The listing builds one solid part. Answer for the finished solid, in the listing's coordinates (mm). A direction names the side the tool comes from. Coordinates: 2 decimals unless noted, no trailing zeros. Write each loop counter-clockwise with the first axis right and the second up, starting at its lowest first coordinate (ties: lowest second). Pieces come first, ordered by that corner, then holes.
from build123d import *

# Parameters (mm, degrees)
SKETCH1_W           = 305
SKETCH1_H           = 305
BOSS_EXTRUDE2_DEPTH = 874
SKETCH3_W           = 100
SKETCH3_H           = 100
BOSS_EXTRUDE4_DEPTH = 100
CUT_EXTRUDE3_DEPTH  = 100
SKETCH8_W           = 305
SKETCH8_H           = 305
BOSS_EXTRUDE5_DEPTH = 66


with BuildPart() as part:
    # Sketch1 → Boss-Extrude2 (new body)
    with BuildSketch(Plane.XY):
        with Locations((152.5, 152.5)):
            Rectangle(SKETCH1_W, SKETCH1_H)
    extrude(amount=BOSS_EXTRUDE2_DEPTH)

    # Sketch3 → Boss-Extrude4 (add)
    with BuildSketch(Plane.ZY):
        with Locations((774, 152.5)):
            Rectangle(SKETCH3_W, SKETCH3_H)
    extrude(amount=BOSS_EXTRUDE4_DEPTH)

    # Sketch5 → Cut-Extrude3 (cut)
    with BuildSketch(Plane.XZ.offset(-102.5)):
        Polygon((-100, 824), (0, 824), (-100, 724), align=None)
    extrude(amount=-CUT_EXTRUDE3_DEPTH, mode=Mode.SUBTRACT)

    # Sketch2 → Cut-Loft2 section 0
    with BuildSketch(Plane(origin=(0, 0, 0), x_dir=(-1, 0, 0), z_dir=(0, 0, -1))):
        with BuildLine():
            Line((-242.5, 242.5), (-62.5, 242.5))
            Line((-62.5, 242.5), (-62.5, 62.5))
            Line((-62.5, 62.5), (-242.5, 62.5))
            Line((-242.5, 62.5), (-242.5, 242.5))
        make_face()
    # Sketch6 → Cut-Loft2 section 1
    with BuildSketch(Plane.XY.offset(874)):
        with BuildLine():
            Line((22.5, 282.5), (282.5, 282.5))
            Line((282.5, 282.5), (282.5, 22.5))
            Line((282.5, 22.5), (22.5, 22.5))
            Line((22.5, 22.5), (22.5, 282.5))
        make_face()
    loft(mode=Mode.SUBTRACT)

    # Sketch8 → Boss-Extrude5 (add)
    with BuildSketch(Plane(origin=(0, 0, 0), x_dir=(-1, 0, 0), z_dir=(0, 0, -1))):
        with Locations((-152.5, 152.5)):
            Rectangle(SKETCH8_W, SKETCH8_H)
    extrude(amount=BOSS_EXTRUDE5_DEPTH)


solid = part.part
Q1. Find the intervals of material crossed by probe 1 along Y at (x, z) = (154, 632); probe 2 along Y at (x, z) = (113.5, 283); probe 3 along X at (y, z) = (169.5, 466.5), in increasing order.
Answers below:
probe 1: y = 0 to 33.58, 271.42 to 305
probe 2: y = 0 to 49.55, 255.45 to 305
probe 3: x = 0 to 41.15, 263.85 to 305
Q2. The part is cut by section A-A, the plane x = -45.5. Write down the section's boundary in (y, z), then the cut area to 3 significant figures.
Answers below:
outline: (102.5, 724) - (202.5, 724) - (202.5, 778.5) - (102.5, 778.5) - close
area: 5,450 mm2
Q3. Given pin 1 (12 mm diameter, centred on y = 33, z = 400, fed in from -X); pin 2 (10 mm diameter, centred on x = 196, z = 578.5, fed in from -Y); pin 3 (6 mm diameter, centred on x = 159.5, y = 230, fed in from +Z), each flat-ended and moving along its own axis, determine where each tip first touches the part or whether it passes through.
Answers below:
pin 1: stops at x = 0
pin 2: stops at y = 0
pin 3: stops at z = 0
Q4. Determine the mould class of faces 1 (the face through (-38, 202.5, 762)), 2 (the face through (155, 0, 411)), 3 (the face through (154, 154, 0)), 4 (the face through (305, 150, 411)) for opening direction Y: released by +Y, released by -Y, zero draft, split by the parting line, or undercut.
Answers below:
face 1: released by +Y
face 2: released by -Y
face 3: undercut
face 4: zero draft
Q5. Which of the six approach directions +Z, -Z, +X, -X, +Y, -Y give full straight-line access (tool end or side, diameter ignored) to faces 5 (the face through (15, 155, 874)), 6 (the face through (-38, 102.5, 762)), 7 (the face through (-49, 152, 724))?
Answers below:
face 5: +Z, +X, -X, +Y, -Y
face 6: +Z, -Z, -X, -Y
face 7: -Z, -X, +Y, -Y
